from build123d import *

# Parameters (mm, degrees)
SKETCH1_W                 = 6
SKETCH1_H                 = 8
CUT_EXTRUDE1_REACH        = 80.305
CUT_EXTRUDE1_START_RADIUS = 10
CUT_EXTRUDE1_END_RADIUS   = 10
SKETCH2_W                 = 13
SKETCH2_H                 = 2
CIRPATTERN1_COUNT         = 10
SKETCH3_R                 = 10
BOSS_EXTRUDE1_DEPTH       = 10
CHAMFER2_SIZE             = 4
CHAMFER6_SIZE             = 10
CHAMFER6_SIZE2            = 4
CHAMFER3_SIZE             = 4
CHAMFER5_SIZE             = 4
BODY_MOVE_COPY2_ANGLE     = 180
SKETCH5_R                 = 10
BOSS_EXTRUDE2_DEPTH       = 46
BOSS_EXTRUDE3_START       = 52
SKETCH6_R                 = 10
BOSS_EXTRUDE3_DEPTH       = 52
BOSS_EXTRUDE4_START       = 52
SKETCH6_3_R               = 3
BOSS_EXTRUDE4_DEPTH       = 10
FILLET1_R                 = 0.5


with BuildPart() as part:
    # Sketch1 → Revolve1 (revolve)
    with BuildSketch(Plane.YZ, mode=Mode.PRIVATE) as revolve1_sk:
        Polygon((57, 10), (0, 10), (0, 0), (62, 0), (62, 8), align=None)
        with Locations((65, 4)):
            Rectangle(SKETCH1_W, SKETCH1_H)
        Polygon((68, 10), (68, 8), (68, 0), (76, 0), (76, 10), align=None)
    revolve(revolve1_sk.sketch.rotate(Axis((0, -74.081666102, 0), (0, 1, 0)), 180), axis=Axis((0, -74.081666102, 0), (0, 1, 0)))

    # Cut-Extrude1: from a cylinder face, 80.305 long prism both ways, kept between that surface and its translate by the depth
    cut_extrude1_start = Plane(origin=(0, 37.5, 0), z_dir=(0, -1, 0)) * Cylinder(CUT_EXTRUDE1_START_RADIUS, 181.61, mode=Mode.PRIVATE)
    cut_extrude1_end = Plane(origin=(-1, 37.5, 0), z_dir=(0, -1, 0)) * Cylinder(CUT_EXTRUDE1_END_RADIUS, 181.61, mode=Mode.PRIVATE)
    # Sketch2 → Cut-Extrude1 (cut, from a surface)
    with BuildSketch(Plane.YZ, mode=Mode.PRIVATE) as cut_extrude1_sk1:
        with Locations((37.5, 0)):
            Rectangle(SKETCH2_W, SKETCH2_H)
    cut_extrude1_tool1 = extrude(cut_extrude1_sk1.sketch, amount=CUT_EXTRUDE1_REACH, both=True, mode=Mode.PRIVATE)
    cut_extrude1 = ((cut_extrude1_tool1 & cut_extrude1_start) - cut_extrude1_end).solids().sort_by_distance((9.449874, 37.5, 0))[0]
    add(cut_extrude1, mode=Mode.SUBTRACT)

    # CirPattern1: Cut-Extrude1 ×10 about axis
    cirpattern1_axis = Axis((0, 0, 0), (0, 1, 0))
    for i in range(1, CIRPATTERN1_COUNT):
        add(cut_extrude1.rotate(cirpattern1_axis, i * 360 / CIRPATTERN1_COUNT), mode=Mode.SUBTRACT)


with BuildPart() as body_2:
    # Sketch3 → Boss-Extrude1 (new body)
    # profile 1 of 2: a face of its own
    with BuildSketch(Plane.XZ):
        with BuildLine():
            Line((-37.340859119, 14.340859119), (-13, -10))
            Line((-13, -10), (-13, -27))
            ThreePointArc((-13, -27), (0, -40), (13, -27))
            Line((13, -27), (13, -10))
            Line((13, -10), (37.340859119, 14.340859119))
            ThreePointArc((37.340859119, 14.340859119), (0, 40), (-37.340859119, 14.340859119))
        make_face()
        with Locations(Location((0, 0, 0), (0, 0, 270))):
            Circle(SKETCH3_R, mode=Mode.SUBTRACT)
    # profile 2 of 2: a face of its own
    with BuildSketch(Plane.XZ):
        with Locations(Location((0, 0, 0), (0, 0, 270))):
            Circle(SKETCH3_R)
    extrude(amount=BOSS_EXTRUDE1_DEPTH)

    # Chamfer2
    chamfer2_edges = [body_2.edges().sort_by_distance(p)[0] for p in [
        (-13, 0, -18.5),
        (13, 0, -18.5),
        (0, 0, -40),
    ]]
    chamfer(chamfer2_edges, length=CHAMFER2_SIZE)

    # Chamfer6
    chamfer6_edges = [body_2.edges().sort_by_distance(p)[0] for p in [
        (0, 0, 40),
    ]]
    chamfer6_side = [body_2.faces().sort_by_distance(p)[0] for p in [
        (0, 0, 9.789093574),
    ]]
    chamfer(chamfer6_edges, length=CHAMFER6_SIZE, length2=CHAMFER6_SIZE2, reference=chamfer6_side[0])

    # Chamfer3
    chamfer3_edges = [body_2.edges().sort_by_distance(p)[0] for p in [
        (19.162771735, 0, -3.837228265),
    ]]
    chamfer(chamfer3_edges, length=CHAMFER3_SIZE)

    # Chamfer5
    chamfer5_edges = [body_2.edges().sort_by_distance(p)[0] for p in [
        (-19.162771735, 0, -3.837228265),
    ]]
    chamfer(chamfer5_edges, length=CHAMFER5_SIZE)


with BuildPart() as body_3:
    # Body-Move/Copy1: copy of body 2
    add(body_2.part.moved(Location((0, -36, 0))))


with BuildPart() as body_3_1:
    # Body-Move/Copy2: moved
    add(body_3.part.rotate(Axis((0, -51, 0), (0, 0, 1)), BODY_MOVE_COPY2_ANGLE))


with BuildPart() as body_2_1:
    add(body_2.part)

    add(body_3_1.part)  # Boss-Extrude2 merges body 3
    # Sketch5 → Boss-Extrude2 (add)
    with BuildSketch(Plane.XZ.offset(10)):
        with Locations(Location((0, -27, 0), (0, 0, 270))):
            Circle(SKETCH5_R)
    extrude(amount=BOSS_EXTRUDE2_DEPTH)

    # Sketch6 → Boss-Extrude3 (add)
    with BuildSketch(Plane.XZ.offset(66).offset(BOSS_EXTRUDE3_START)):
        with Locations(Location((0, 0, 0), (0, 0, 180))):
            Circle(SKETCH6_R)
    extrude(amount=-BOSS_EXTRUDE3_DEPTH)

    # Sketch6<3> → Boss-Extrude4 (add)
    with BuildSketch(Plane.XZ.offset(66).offset(BOSS_EXTRUDE4_START)):
        Circle(SKETCH6_3_R)
    extrude(amount=BOSS_EXTRUDE4_DEPTH)

    # Fillet1
    fillet1_edges = [body_2_1.edges().sort_by_distance(p)[0] for p in [
        (10, -118, 0),
    ]]
    fillet(fillet1_edges, radius=FILLET1_R)


with BuildPart() as part_1:
    add(part.part)

    # Combine1: union body 2
    add(body_2_1.part)


solid = part_1.part
Can you work these out from the model? Positions are in its coordinate system, mm. A direction names the side the tool comes from. Round coordinates to 2 decimals unless told otherwise and drop trailing zeros. Write each loop counter-clockwise with the first axis right and the second up, starting at its lowest first coordinate (ties: lowest second). Pieces come first, ordered by that corner, then holes. Notation, with made-up numbers: M -26,30.5 L -6,30.5 A19 ccw -6,58.5 Z; hole C 87.5,-19.5 d2. An arc over 180 degrees is marked long. Use CSV: the item, a comma, the result in double quotes.
(1) We'd pull the mould along Y, two halves only. Please class faces 1 (the flat face through (0, -128, 0)), 2 (the cylindrical face through (10, -92, 0)), 3 (the cylindrical face through (3, -32.68, -36.54)): +Y half, -Y half, draft (parallel to the pull), parting line (faces both ways), or undercut.
Check values:
face 1,"-Y half"
face 2,"draft"
face 3,"undercut"
(2) Imagine slicing it at A-A (z = -13). Write out the boundary of the cut face in (x, y).
Check values:
outline,"M -13,-62 L -9,-66 L 9,-66 L 13,-62 L 13,-56 L -13,-56 Z; M -13,-10 L 13,-10 L 13,-4 L 9,0 L -9,0 L -13,-4 Z"
(3) On a 3-axis mill with a long thin cutter (end or side, diameter ignored), from which of +Z, -Z, +X, -X, +Y, -Y can I reach the whole of each face in a straight line? I mean faces 4 (the cylindrical face through (0, 72, 10)), 5 (the flat face through (-8.2, 68, 0)), 6 (the flat face through (11, -2, -18)), 7 (the cylindrical face through (0, -59, -40)). Say none if no direction works.
Check values:
face 4,"+Y"
face 5,"none"
face 6,"-Z, +X, +Y"
face 7,"-Z, +Y, -Y"
(4) I'm going to push flat-ended pins straight in: pin 1 (1.8 mm diameter, centred on y = -59, z = -19, fed in from -X); pin 2 (10 mm diameter, centred on x = -25.5, z = 17.5, fed in from +Y); pin 3 (6 mm diameter, centred on x = 26.5, z = 15.5, fed in from -Y). Where does each tip first touch, or does it pass through?
Check values:
pin 1,"x = -13"
pin 2,"y = 0"
pin 3,"y = -66"
(5) Imagine slicing it at B-B (y = -84.5). Write out the boundary of the cut face in (x, z).
Check values:
outline,"C 0,0 d20"
(6) I need wall thicknesses on line 1 along Y through (x, z) = (-3, 12.5); line 2 along X through (y, z) = (23, 2); line 3 along Z through (x, y) = (7.5, -100.5). Which ranges of each line are inside material? Lowest first, please.
Check values:
line 1,"-66 to -56, -10 to 0"
line 2,"-9.8 to 9.8"
line 3,"-6.61 to 6.61"
